```python
from build123d import *

# Parameters (mm, degrees)
SKETCH1_W                 = 32.5
SKETCH1_H                 = 42
BOSS_EXTRUDE2_DEPTH       = 5
F_2_56_TAPPED_HOLE1_D     = 1.778
F_2_56_TAPPED_HOLE1_DEPTH = 7.46583491
F_2_56_TAPPED_HOLE1_TIP   = 0.53416509
F_2_56_TAPPED_HOLE2_D     = 1.778
F_2_56_TAPPED_HOLE2_DEPTH = 7.46583491
F_2_56_TAPPED_HOLE2_TIP   = 0.53416509
CUT_EXTRUDE1_DEPTH        = 5


with BuildPart() as part:
    # Sketch1 → Boss-Extrude2 (new body)
    with BuildSketch(Plane.XY):
        with Locations((16.25, 21)):
            Rectangle(SKETCH1_W, SKETCH1_H)
    extrude(amount=BOSS_EXTRUDE2_DEPTH)

    # #2-56 Tapped Hole1
    with Locations(Plane.ZY):
        with Locations((2.5, 34), (2.5, 8)):
            Hole(F_2_56_TAPPED_HOLE1_D / 2, depth=F_2_56_TAPPED_HOLE1_DEPTH)
            with Locations((0, 0, -(F_2_56_TAPPED_HOLE1_DEPTH + F_2_56_TAPPED_HOLE1_TIP / 2))):  # 118° drill point
                Cone(0, F_2_56_TAPPED_HOLE1_D / 2, F_2_56_TAPPED_HOLE1_TIP, mode=Mode.SUBTRACT)

    # #2-56 Tapped Hole2
    with Locations(Plane(origin=(32.5, 0, 0), x_dir=(0, 0, -1), z_dir=(1, 0, 0))):
        with Locations((-2.5, 34), (-2.5, 8)):
            Hole(F_2_56_TAPPED_HOLE2_D / 2, depth=F_2_56_TAPPED_HOLE2_DEPTH)
            with Locations((0, 0, -(F_2_56_TAPPED_HOLE2_DEPTH + F_2_56_TAPPED_HOLE2_TIP / 2))):  # 118° drill point
                Cone(0, F_2_56_TAPPED_HOLE2_D / 2, F_2_56_TAPPED_HOLE2_TIP, mode=Mode.SUBTRACT)

    # Sketch9 → Cut-Extrude1 (cut)
    with BuildSketch(Plane(origin=(0, 0, 0), x_dir=(-1, 0, 0), z_dir=(0, 0, -1))):
        with BuildLine():
            ThreePointArc((-15.1, 21), (-12.1, 18), (-9.1, 21))
            Line((-9.1, 21), (-12.1, 21))
            Line((-12.1, 21), (-15.1, 21))
        make_face()
        with BuildLine():
            Line((-12.1, 21), (-9.1, 21))
            ThreePointArc((-9.1, 21), (-12.1, 24), (-15.1, 21))
            Line((-15.1, 21), (-12.1, 21))
        make_face()
    extrude(amount=-CUT_EXTRUDE1_DEPTH, mode=Mode.SUBTRACT)


solid = part.part
```
Here's how the part is built. I have some questions about the finished solid (model axes, mm). A direction names the side the tool comes from. Coordinates: 2 decimals unless noted, no trailing zeros. Order: outer loops, then holes, each group sorted by start corner. A loop starts at its lowest first (then second) coordinate and runs counter-clockwise, first axis right, second up. Notation, with made-up numbers: M 14,-3.5 L 43,-3.5 A14 ccw 43,6.5 Z; hole C 26,64 d3. An arc over 180 degrees is marked long. Answer as a JSON object with one key per item and string values. Group by question number.
(1) Suppose I cut it at C-C, the plane x = 3. Please give me the cut outline in (y, z), then the cut area to 3 significant figures.
(2) I need wall thicknesses on probe 1 along Y at (x, z) = (6, 2.5); probe 2 along Y at (x, z) = (26, 1.85); probe 3 along Y at (x, z) = (12.1, 2.7). Which ranges of each line are inside material? Lowest first, please.
(3) If we mould it in two halves opening along Y, with no side actions, what happens to faces 4 (the face through (16, 42, 2)), 5 (the face through (28.71, 7.13, 2.31)), 6 (the face through (16, 21, 0))? For each: released by +Y, released by -Y, zero draft, split by the parting line, or undercut.
(4) For pin 1 (1.4 mm diameter, centred on y = 34, z = 2.5, fed in from +X), with a flat end and sliding along its axis, tell me the tip position at first contact or that it passes through.
(5) Which directions (+Z, -Z, +X, -X, +Y, -Y) give clear straight access to the entire face, cutting with the end or side of a thin tool? Please do faces 1 (the face through (16, 21, 5)), 2 (the face through (3.79, 33.21, 2.09)), 3 (the face through (28.71, 33.13, 2.31)).
(6) Suppose I cut it at B-B, the plane x = 12.1. Please give me the cut outline in (y, z).
(7) Suppose I cut it at A-A, the plane y = 21. Please give me the cut outline in (x, z), then the cut area to 4 significant figures.
Values found:
{
 "1": {"outline": "M 0,0 L 42,0 L 42,5 L 0,5 Z; hole C 8,2.5 d1.78; hole C 34,2.5 d1.78", "area": "205 mm^2"},
 "2": {"probe 1": "y = 0 to 7.11, 8.89 to 33.11, 34.89 to 42", "probe 2": "y = 0 to 7.39, 8.61 to 33.39, 34.61 to 42", "probe 3": "y = 0 to 18, 24 to 42"},
 "3": {"face 4": "released by +Y", "face 5": "undercut", "face 6": "zero draft"},
 "4": {"pin 1": "stops at x = 24.92"},
 "5": {"face 1": "+Z, +X, -X, +Y, -Y", "face 2": "-X", "face 3": "+X"},
 "6": {"outline": "M 0,0 L 18,0 L 18,5 L 0,5 Z; M 24,0 L 42,0 L 42,5 L 24,5 Z"},
 "7": {"outline": "M 0,0 L 9.1,0 L 9.1,5 L 0,5 Z; M 15.1,0 L 32.5,0 L 32.5,5 L 15.1,5 Z", "area": "132.5 mm^2"}
}
